The model under review builds one solid part; all positions refer to its coordinate system, in mm. A direction names the side the tool comes from. Coordinates: 2 decimals unless noted, no trailing zeros. Loops run counter-clockwise (first coordinate to the right, second up) from the corner with the lowest first, then second, coordinate; pieces in that order, holes last. Notation, with made-up numbers: M -39.75,44.25 L 17.25,44.25 A13 cw 17.25,65.25 Z; hole C -13,64 d3. An arc over 180 degrees is marked long. Return JSON: item names as keys, results as strings.
Autodesk Fusion 360 part; units mm, degrees
sketch "Sketch1" plane through (0, 0, 0) normal (0, 0, 1) x (1, 0, 0) in component "LightSwitchShelf"
  line L0 (0, 0) -> (93.15, 0)
  line L1 (93.15, 0) -> (93.15, 3)
  line L2 (93.15, 3) -> (0, 3)
  line L3 (0, 3) -> (0, 0)
  line L4 (0, 3) -> (5, 3)
  line L5 (93.15, 3) -> (88.15, 3)
  line L6 (46.575, 3) -> (46.575, 86.15) construction
  line L7 (0.5, 86.15) -> (46.575, 86.15) construction
  line L8 (46.575, 86.15) -> (92.65, 86.15) construction
  line L9 (0.5, 86.15) -> (5.5, 86.15)
  line L10 (92.65, 86.15) -> (87.65, 86.15)
  line L11 (0.5, 86.15) -> (0, 3)
  line L12 (5, 3) -> (5.5, 86.15)
  line L13 (87.65, 86.15) -> (88.15, 3)
  line L14 (93.15, 3) -> (92.65, 86.15)
  line L15 (0.5, 86.15) -> (9.4998, 86.0959)
  line L16 (0.5, 86.15) -> (0.518, 89.1499)
  line L17 (0.518, 89.1499) -> (9.4998, 86.0959)
  line L18 (92.65, 86.15) -> (83.6502, 86.0959)
  line L19 (92.65, 86.15) -> (92.65, 89.15)
  line L20 (92.65, 89.15) -> (83.6502, 86.0959)
  dimension "d2" = 3
  dimension "d8" = 5
  dimension "d10" = 83.15
  dimension "d11" = 46.075
  dimension "d14" = 9
  dimension "d15" = 3
  dimension "d17" = 3
  dimension "d18" = 90
  dimension "d19" = 90
  dimension "d29" = 83.15
  dimension "d30" = 82.15
extrude "Extrude1" add sketch "Sketch1" along normal blind 3 makes body 1 in component "LightSwitchShelf"
extrude "Extrude2" add sketch "Sketch1" along normal blind 55 separate body contours L0 L1 L2 L3 L4 L5 makes body 2 in component "LightSwitchShelf"
sketch "Sketch2" plane through (0, 0, 0) normal (0, -1, 0) x (1, 0, 0) in component "LightSwitchShelf"
  line L0 (0, 0) -> (93.15, 0)
  line L1 (93.15, 0) -> (93.15, 55)
  line L2 (93.15, 55) -> (0, 55)
  line L3 (0, 55) -> (0, 0)
  line L4 (46.575, 55) -> (46.575, 0) construction
  line L5 (0, 27.5) -> (93.15, 27.5) construction
  line L6 (88.075, 3.5) -> (5.075, 3.5)
  line L7 (5.075, 3.5) -> (5.075, 51.5)
  line L8 (5.075, 51.5) -> (88.075, 51.5)
  line L9 (88.075, 51.5) -> (88.075, 3.5)
  line L10 (88.075, 3.5) -> (5.075, 51.5) construction
  line L11 (5.075, 3.5) -> (88.075, 51.5) construction
  point P0 (46.575, 27.5)
  dimension "d24" = 48
  dimension "d25" = 83
extrude "Extrude3" add sketch "Sketch2" along normal blind 2 bodies 1 2 in component "LightSwitchShelf"
chamfer "Chamfer1" distance 2 angle 45 4 edges at (5.075, -2, 27.5) (46.575, -2, 51.5) (88.075, -2, 27.5) (46.575, -2, 3.5) on bodies 1 in component "LightSwitchShelf"
fillet "Fillet1" radius 2.5 2 edges at (0, 0.5, 55) (93.15, 0.5, 55) on bodies 1 in component "LightSwitchShelf"
component "LightSwitchShelf" placed x (1, 0, 0) y (0, 1, 0) z (0, 0, 1) at (0, 0, 0)
equation "d11 = ( 83.15 / 2 ) * 1 mm + 4.5 mm"
1. The part is to be moulded in two halves that separate along X. For faces 1 (the face through (0, 1, 26)), 2 (the face through (3, 47, 3)), 3 (the face through (46, 0, 27)), 4 (the face through (88.213, 87.644, 1.479)), say which applies: released by +X, released by -X, zero draft, split by the parting line, or undercut.
Check values:
{"face 1": "released by -X", "face 2": "zero draft", "face 3": "undercut", "face 4": "undercut"}
2. Add section B-B on y = 70. Give the boundary of the cut face in (x, z).
Check values:
{"outline": "M 0.4,0 L 5.4,0 L 5.4,3 L 0.4,3 Z; M 87.75,0 L 92.75,0 L 92.75,3 L 87.75,3 Z"}
3. To check wall thickness, follow line 1 (Y direction, x = 76, z = 14); line 2 (Y direction, x = 38.5, z = 52). State the ranges of each line that lie inside material, in increasing order.
Check values:
{"line 1": "0 to 3", "line 2": "-0.5 to 3"}
4. Insertion check: pin 1 Ø14.5 at (x, z) = (50.5, 39) entering from -Y; pin 2 Ø3 at (x, y) = (88, 49.5) entering from +Z; pin 3 Ø12 at (x, y) = (13.5, 29) entering from -Z; pin 4 Ø2.5 at (y, z) = (87, 2) entering from +X. Each pin has a flat end and moves straight along its axis. Give the tip position at first contact, or say it passes through.
Check values:
{"pin 1": "y = 0", "pin 2": "z = 3", "pin 3": "through", "pin 4": "x = 92.65"}
5. Machinability: for faces 5 (the face through (92.65, 88, 1)), 6 (the face through (4.946, 87.644, 1.479)), 7 (the face through (5, 34, 0)), which of the approach directions +Z, -Z, +X, -X, +Y, -Y give a long, thin tool a straight path to every point of the face, cutting with its end or side? Answer none if there is none.
Check values:
{"face 5": "+Z, -Z, +X, +Y", "face 6": "+Z, -Z, +Y", "face 7": "-Z, +X, -X, +Y, -Y"}
